Could you check a few things on this model? Use its own coordinates, in mm. A direction names the side the tool comes from. Round coordinates to 2 decimals unless told otherwise and drop trailing zeros. Loops run counter-clockwise (first coordinate to the right, second up) from the corner with the lowest first, then second, coordinate; pieces in that order, holes last.
from build123d import *

# Parameters (mm, degrees)
SKETCH_W      = 72
SKETCH_H      = 53
PAD_DEPTH     = 2.5
SKETCH001_R   = 4
PAD001_DEPTH  = 6
SKETCH002_R   = 1.9
HOLE_DEPTH    = 6
SKETCH003_R   = 1.6
HOLE001_DEPTH = 2.501
SKETCH004_R   = 4
PAD002_DEPTH  = 18
SKETCH005_R   = 1.9
HOLE002_DEPTH = 6


with BuildPart() as part:
    # Sketch → Pad (new body)
    with BuildSketch(Plane.XY):
        Rectangle(SKETCH_W, SKETCH_H)
    extrude(amount=PAD_DEPTH)

    # Sketch001 (on Face6 of Pad) → Pad001 (join)
    with BuildSketch(Plane.XY.offset(2.5)):
        with Locations((-22, 18.45)):
            Circle(SKETCH001_R)
        with Locations((22, 18.45)):
            Circle(SKETCH001_R)
        with Locations((-22, -18.45)):
            Circle(SKETCH001_R)
        with Locations((22, -18.45)):
            Circle(SKETCH001_R)
    extrude(amount=PAD001_DEPTH)

    # Sketch002 (on Face14 of Pad001) → Hole (cut)
    with BuildSketch(Plane.XY.offset(8.5)):
        with Locations((-22, 18.45)):
            Circle(SKETCH002_R)
        with Locations((22, 18.45)):
            Circle(SKETCH002_R)
        with Locations((-22, -18.45)):
            Circle(SKETCH002_R)
        with Locations((22, -18.45)):
            Circle(SKETCH002_R)
    extrude(amount=-HOLE_DEPTH, mode=Mode.SUBTRACT)

    # Sketch003 (on Face5 of Hole) → Hole001 (cut, through all)
    with BuildSketch(Plane.XY.offset(2.5)):
        with Locations((-29.2, 21)):
            Circle(SKETCH003_R)
        with Locations((-29.2, -21)):
            Circle(SKETCH003_R)
        with Locations((29.2, 21)):
            Circle(SKETCH003_R)
        with Locations((29.2, -21)):
            Circle(SKETCH003_R)
    extrude(amount=-HOLE001_DEPTH, mode=Mode.SUBTRACT)

    # Sketch004 (on Face5 of Hole001) → Pad002 (join)
    with BuildSketch(Plane.XY.offset(2.5)):
        with Locations((30, 5)):
            Circle(SKETCH004_R)
        with Locations((-30, -5)):
            Circle(SKETCH004_R)
    extrude(amount=PAD002_DEPTH)

    # Sketch005 (on Face19 of Pad002) → Hole002 (cut)
    with BuildSketch(Plane.XY.offset(20.5)):
        with Locations((-30, -5)):
            Circle(SKETCH005_R)
        with Locations((30, 5)):
            Circle(SKETCH005_R)
    extrude(amount=-HOLE002_DEPTH, mode=Mode.SUBTRACT)


solid = part.part
Item 1: If we section it at A-A, the plane z = 7.75: Count the separate pieces of the cut face and the enclosed holes in it, then the cut area to 3 significant figures.
Results list:
separate pieces: 6
enclosed holes: 4
area: 256 mm2
Item 2: Will these pins go through, and if not, where does the flat tip stop? pin 1 (2.5 mm diameter, centred on x = 23.5, y = 19, fed in from +Z); pin 2 (4 mm diameter, centred on y = 11.5, z = 5.5, fed in from -X); pin 3 (2 mm diameter, centred on x = 28.5, z = 8.5, fed in from -Y); pin 4 (3.5 mm diameter, centred on x = -22, y = -18.45, fed in from +Z).
Results list:
pin 1: stops at z = 8.5
pin 2: passes through
pin 3: stops at y = 1.03
pin 4: stops at z = 2.5
Item 3: For faces 4 (the flat face through (22, -18, 2.5)), 5 (the flat face through (-28, -6, 20.5)), which set-ups out of +Z, -Z, +X, -X, +Y, -Y let a thin tool reach every point of the face, with its end or its side?
Results list:
face 4: +Z
face 5: +Z, +X, -X, +Y, -Y
Item 4: We'd pull the mould along X, two halves only. Please class faces 1 (the flat face through (24, -19, 8.5)), 2 (the flat face through (-36, 0, 1)), 3 (the flat face through (-30, -5, 14.5)): released by +X, released by -X, zero draft, split by the parting line, or undercut.
Results list:
face 1: zero draft
face 2: released by -X
face 3: undercut
Item 5: If we section it at C-C, the plane x = 22: Please give me the cut outline in (y, z).
Results list:
outline: (-26.5, 0) - (26.5, 0) - (26.5, 2.5) - (22.45, 2.5) - (22.45, 8.5) - (20.35, 8.5) - (20.35, 2.5) - (16.55, 2.5) - (16.55, 8.5) - (14.45, 8.5) - (14.45, 2.5) - (-14.45, 2.5) - (-14.45, 8.5) - (-16.55, 8.5) - (-16.55, 2.5) - (-20.35, 2.5) - (-20.35, 8.5) - (-22.45, 8.5) - (-22.45, 2.5) - (-26.5, 2.5) - close
Item 6: If I drill on line 1 along Y through (x, z) = (-30, 19); line 2 along Y through (x, z) = (29.2, 1.4); line 3 along Z through (x, y) = (23.5, 7), over which ranges is the centre line in solid material (lowest first)?
Results list:
line 1: y = -9 to -6.9, -3.1 to -1
line 2: y = -26.5 to -22.6, -19.4 to 19.4, 22.6 to 26.5
line 3: z = 0 to 2.5
Item 7: If we section it at B-B, the plane y = 18.45: Please give me the cut outline in (x, z).
Results list:
outline: (-36, 0) - (36, 0) - (36, 2.5) - (26, 2.5) - (26, 8.5) - (23.9, 8.5) - (23.9, 2.5) - (20.1, 2.5) - (20.1, 8.5) - (18, 8.5) - (18, 2.5) - (-18, 2.5) - (-18, 8.5) - (-20.1, 8.5) - (-20.1, 2.5) - (-23.9, 2.5) - (-23.9, 8.5) - (-26, 8.5) - (-26, 2.5) - (-36, 2.5) - close
Item 8: If we section it at D-D, the plane z = 16: Please give me the cut outline in (x, y), then the cut area to 3 significant figures.
Results list:
outline: circle Ø8 at (-30, -5); circle Ø8 at (30, 5); hole circle Ø3.8 at (-30, -5); hole circle Ø3.8 at (30, 5)
area: 77.8 mm2
